Source: three-view drawing plus pictorial views. Frame: mm from the lowest corner of the part. A direction names the side the tool comes from. Coordinates: 2 decimals unless noted, no trailing zeros. Write each loop counter-clockwise with the first axis right and the second up, starting at its lowest first coordinate (ties: lowest second). Pieces come first, ordered by that corner, then holes. Notation, with made-up numbers: (-15, 5.5) - (14, 5.5) arc R25 ccw to (14, 35.5) - close; hole circle Ø6 at (69.25, -37). An arc over 180 degrees is marked (long way). Answer as a JSON object with one key per item and string values. Group by question number.
Item 1: Mould query, pull axis X, two halves, no side actions, for the marked faces 1, 2 and 3. Classes: pulls with the +X half, pulls with the -X half, needs draft (parallel to the pull), parting line crosses it, or undercut.
Item 2: Line query: line 1 along Y through (x, z) = (3.15, 25.4); line 2 along Y through (x, z) = (17.5, 30) (1 decimal); line 3 along X through (y, z) = (35, 22) (1 decimal). Output: solid intervals per line, ascending. Write a range as from..to.
Item 3: Section C-C on y = 7. Return loops of the section in (x, z) (1 decimal).
Item 4: Section D-D on x = 16.5. Return loops of the section in (y, z), and give its area (3 significant figures).
Item 5: Section A-A on z = 25.4. State how many separate pieces and enclosed holes the cut face has.
Item 6: Set-up query: the marked faces 4, 5 and 6. Return all of +Z, -Z, +X, -X, +Y, -Y with unobstructed straight access to the full face (end or side cutting, diameter ignored); none if empty.
Item 7: First-contact query: pin 1 Ø1.5 at (x, z) = (7.5, 17) entering from +Y; pin 2 Ø1.4 at (x, z) = (2, 8) entering from -Y; pin 3 Ø12 at (x, y) = (18.5, 17) entering from -Z; pin 4 Ø8 at (y, z) = (41.275, 25.4) entering from +X. Flat tips, straight axial feed; report the tip coordinate or a pass-through.
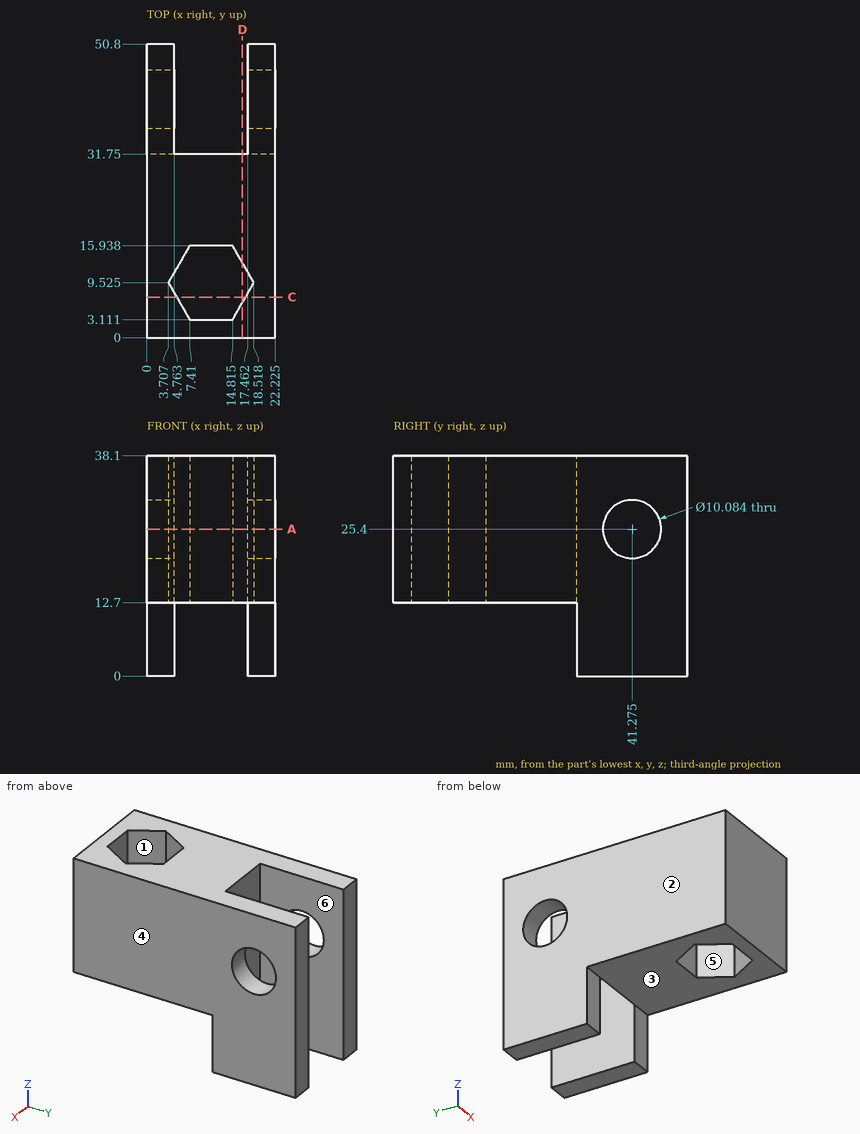
Checks:
{
 "1": {"face 1": "undercut", "face 2": "pulls with the -X half", "face 3": "needs draft"},
 "2": {"line 1": "0..36.23, 46.32..50.8", "line 2": "0..7.8, 11.3..39.2, 43.3..50.8", "line 3": "0..4.8, 17.5..22.2"},
 "3": {"outline": "(0, 12.7) - (5.2, 12.7) - (5.2, 38.1) - (0, 38.1) - close; (17.1, 12.7) - (22.2, 12.7) - (22.2, 38.1) - (17.1, 38.1) - close"},
 "4": {"outline": "(0, 12.7) - (6.03, 12.7) - (6.03, 38.1) - (0, 38.1) - close; (13.02, 12.7) - (31.75, 12.7) - (31.75, 38.1) - (13.02, 38.1) - close", "area": "629 mm^2"},
 "5": {"separate pieces": "3", "enclosed holes": "1"},
 "6": {"face 4": "+Z, -Z, +X, +Y, -Y", "face 5": "+Z, -Z", "face 6": "+Z, -Z, +Y"},
 "7": {"pin 1": "y = 31.75", "pin 2": "y = 31.75", "pin 3": "z = 12.7", "pin 4": "through"}
}
